Could you check a few things on this drawing? It's one solid part, dimensions in mm from its lowest x, y, z. A direction names the side the tool comes from. Coordinates: 2 decimals unless noted, no trailing zeros. Order: outer loops, then holes, each group sorted by start corner. A loop starts at its lowest first (then second) coordinate and runs counter-clockwise, first axis right, second up.
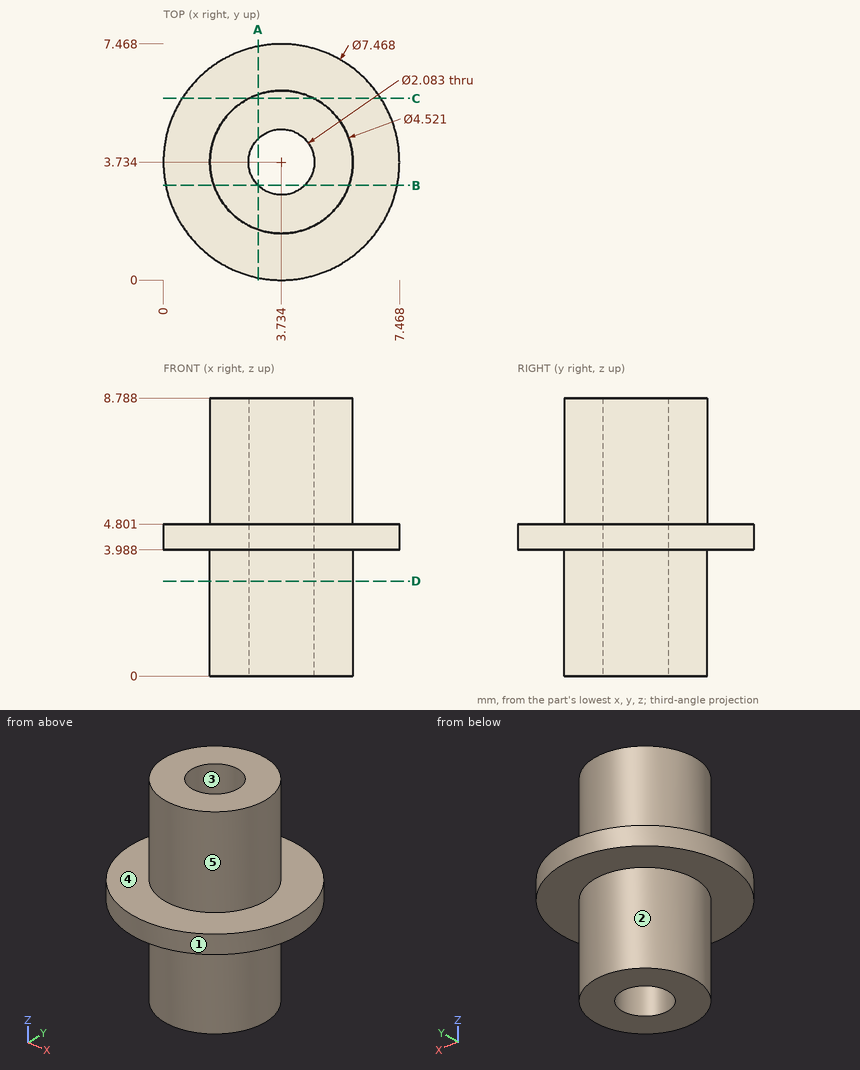
1. I'm going to push flat-ended pins straight in: pin 1 (4 mm diameter, centred on y = 3, z = 6.5, fed in from +X); pin 2 (1.2 mm diameter, centred on x = 3.73, y = 3.73, fed in from +Z); pin 3 (4 mm diameter, centred on x = 6, z = 4, fed in from +Y). Where does each tip first touch, or does it pass through?
Completed:
pin 1: stops at x = 7.47
pin 2: passes through
pin 3: stops at y = 7.46
2. Imagine slicing it at D-D on z = 3. Please give me the cut outline in (x, y) (1 decimal).
Completed:
outline: circle Ø4.5 at (3.7, 3.7); hole circle Ø2.1 at (3.7, 3.7)
3. Please list where these lines run through material, in increasing order: probe 1 along Y at (x, z) = (3.75, 3.25) (1 decimal); probe 2 along Z at (x, y) = (1.5, 4.5); probe 3 along X at (y, z) = (4.5, 8) (1 decimal).
Completed:
probe 1: y = 1.5 to 2.7, 4.8 to 6
probe 2: z = 3.99 to 4.8
probe 3: x = 1.6 to 3, 4.4 to 5.9
4. On a 3-axis mill with a long thin cutter (end or side, diameter ignored), from which of +Z, -Z, +X, -X, +Y, -Y can I reach the whole of each face in a straight line? I mean the marked faces 1 and 2. Say none if no direction works.
Completed:
face 1: +Z, -Z
face 2: -Z
5. Thinking about a two-plate mould opening in Y: for the marked faces 3, 4 and 5, which applies, pulls with the +Y half, pulls with the -Y half, needs draft (parallel to the pull), parting line crosses it, or undercut?
Completed:
face 3: undercut
face 4: needs draft
face 5: parting line crosses it
6. Imagine slicing it at C-C on y = 5.75. Please give me the cut outline in (x, z), then the cut area to 3 significant figures.
Completed:
outline: (0.59, 3.99) - (2.71, 3.99) - (2.71, 0) - (4.76, 0) - (4.76, 3.99) - (6.88, 3.99) - (6.88, 4.8) - (4.76, 4.8) - (4.76, 8.79) - (2.71, 8.79) - (2.71, 4.8) - (0.59, 4.8) - close
area: 21.4 mm2
7. Imagine slicing it at A-A on x = 3. Please give me the cut outline in (y, z) (1 decimal).
Completed:
outline: (0.1, 4) - (1.6, 4) - (1.6, 0) - (3, 0) - (3, 8.8) - (1.6, 8.8) - (1.6, 4.8) - (0.1, 4.8) - close; (4.5, 0) - (5.9, 0) - (5.9, 4) - (7.4, 4) - (7.4, 4.8) - (5.9, 4.8) - (5.9, 8.8) - (4.5, 8.8) - close
